Geometry check sheet. Reference: the model listing, model coordinates, mm. Face numbers are marked on the shaded views. A direction names the side the tool comes from. Round coordinates to 2 decimals unless told otherwise and drop trailing zeros. Write each loop counter-clockwise with the first axis right and the second up, starting at its lowest first coordinate (ties: lowest second). Pieces come first, ordered by that corner, then holes. Notation, with made-up numbers: M -8,77 L 12,77 A17 cw 12,105 Z; hole C -17,76.25 d11. An arc over 180 degrees is marked long. Put each result on its own line as item: value. Start each with the question number.
(1) Section check C-C on y = -9. Record the cut outline in (x, z) (3 decimals), then the cut area to 3 significant figures.
(2) Material ranges on probe 1 along Y at (x, z) = (16.5, 1.7); probe 2 along Y at (x, z) = (25.5, 2.95); probe 3 along Y at (x, z) = (29, 2), recorded low to high.
(3) Section check A-A on x = 17.5. Record the cut outline in (y, z) (1 decimal).
(4) Gauge pin test, flat ends, axial feed: pin 1 (1.6 mm diameter, centred on x = 22, z = 1.5, fed in from +Y); pin 2 (1.6 mm diameter, centred on x = -13.5, y = 16.5, fed in from -Z). Record the tip position at first contact, or that the pin passes through.
(5) Section check B-B on y = 6.35. Record the cut outline in (x, z) (3 decimals).
(6) Section check D-D on x = 10.5. Record the cut outline in (y, z) (3 decimals).
(7) Mould release check, pull along Y, two halves, no side actions. Record for the marked faces 4, 5 and 6: pulls with the +Y half, pulls with the -Y half, needs draft (parallel to the pull), parting line crosses it, or undercut.
(8) Tool access check on the marked faces 1, 2 and 3. Record the directions out of +Z, -Z, +X, -X, +Y, -Y that give a thin tool (end or side, any length) a straight path to the whole face; none if there is none.
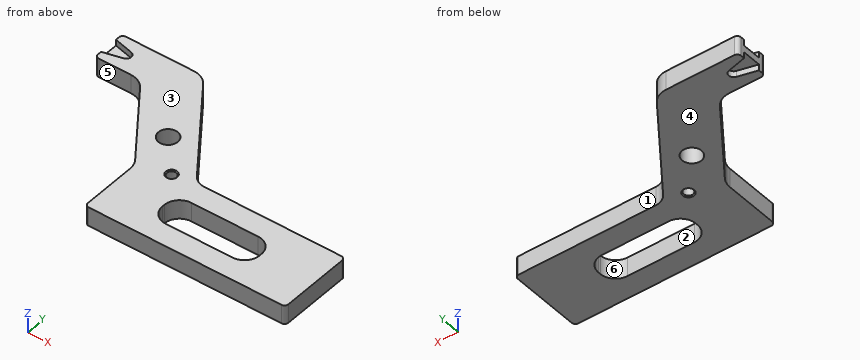
Autodesk Inventor part; units mm, degrees
ref_plane "Work Plane1" through (0, 0, 1.5875) normal (0, 0, 1) x (1, 0, 0)
ref_plane "YZ Plane" through (0, 0, 0) normal (1, 0, 0) x (0, 1, 0)
sketch "Sketch1" plane through (0, 0, 0) normal (0, 0, 1) x (1, 0, 0)
  line L0 (-20.447, 0) -> (20.447, 0)
  line L1 (0, -17.526) -> (0, 25.146)
  line L2 (14.605, -11.43) -> (-14.605, -11.43)
  line L3 (-14.605, -11.43) -> (-14.605, 19.05)
  line L4 (-14.605, 19.05) -> (14.605, 19.05)
  line L5 (14.605, 19.05) -> (14.605, -11.43)
  line L6 (-14.605, 16.6688) -> (-14.605, 19.05)
  point P0 (0, 0)
  dimension "d0" = 29.21
  dimension "d1" = 30.48
  dimension "d2" = 14.605
  dimension "d232" = 19.05
extrude "Extrusion2" add sketch "Sketch1" along normal blind 3.175
sketch "Sketch2" plane through (0, 0, 3.175) normal (0, 0, 1) x (1, 0, 0)
  line L0 (-14.605, -11.43) -> (-14.605, 19.05)
  line L1 (-14.605, 17.78) -> (-11.43, 16.9862)
  line L2 (-11.43, 16.9862) -> (-11.43, 15.3987)
  line L3 (-11.43, 15.3987) -> (-14.605, 14.605)
  line L4 (-14.605, 17.78) -> (-14.605, 14.605)
  line L5 (-14.605, 17.78) -> (-14.605, 19.05)
  arc A0 (-11.43, 15.3987) -> (-11.43, 16.9862) centre (-11.6284, 16.1925) ccw
  point P0 (0, 0)
  dimension "d21" = 3.175
  dimension "d22" = 1.5875
  dimension "d23" = 1.27
  dimension "d66" = 3.175
extrude "Extrusion3" cut sketch "Sketch2" against normal blind 1.016
sketch "Sketch11" plane through (0, 0, 3.175) normal (0, 0, 1) x (1, 0, 0)
  line L0 (14.605, -11.43) -> (-14.605, -11.43)
  line L1 (14.605, 1.27) -> (14.605, 19.05)
  line L2 (-14.605, 13.335) -> (-6.985, 13.335)
  line L3 (-6.985, 13.335) -> (3.175, -0.8164)
  line L4 (10.795, -11.43) -> (-14.605, -11.43)
  line L5 (14.605, 19.05) -> (14.605, -11.43)
  line L6 (14.605, 1.27) -> (11.8393, 1.27)
  line L7 (11.8393, 1.27) -> (-0.9259, 19.05)
  line L8 (-0.9259, 19.05) -> (14.605, 19.05)
  line L9 (-14.605, 13.335) -> (-14.605, -11.43)
  line L10 (3.175, -0.8164) -> (3.175, -11.43)
  point P0 (0, 0)
  point P1 (0, -11.43)
  dimension "d220" = 7.62
  dimension "d221" = 25.4
  dimension "d226" = 12.7
  dimension "d230" = 8.255
  dimension "d263" = 7.62
  dimension "d264" = 54.324
extrude "Extrusion10" cut sketch "Sketch11" against normal through all
sketch "Sketch12" plane through (0, 0, 3.175) normal (0, 0, 1) x (1, 0, 0)
  line L0 (-14.605, 19.05) -> (14.605, 19.05)
  line L1 (-14.605, -11.43) -> (-14.605, 19.05)
  line L2 (-0.2249, 19.05) -> (-2.4073, 19.05)
  line L3 (-0.2419, 3.9428) -> (6.4638, 8.7572)
  line L4 (-0.2419, 3.9428) -> (3.111, 6.35)
  line L5 (3.111, 6.35) -> (6.4638, 8.7572)
  line L6 (-6.985, 13.335) -> (3.175, -0.8164)
  line L7 (11.8393, 1.27) -> (-0.9259, 19.05)
  line L8 (0, 25.146) -> (0, -17.526)
  line L9 (-20.447, 0) -> (20.447, 0)
  point P0 (-14.605, 14.605)
  point P1 (10.795, -11.43)
  dimension "d231" = 6.35
hole "Hole9" at (3.111, 6.35, 3.175) direction (0, 0, -1) diameter 3.2512 end through all
sketch "Sketch16" plane through (14.605, -11.43, 3.175) normal (1, 0, 0) x (0, 0, -1)
  line L0 (3.175, 12.7) -> (0, 12.7)
  line L1 (0, 12.7) -> (0, 0)
  line L2 (3.175, 12.7) -> (3.175, 0)
  line L3 (3.175, 0) -> (0, 0)
  line L4 (0, 12.7) -> (3.175, 12.7)
  line L5 (3.175, 12.7) -> (3.175, 0)
  line L6 (3.175, 0) -> (0, 0)
  line L7 (0, 0) -> (0, 12.7)
extrude "Extrusion14" add sketch "Sketch16" along normal blind 22.098
hole "Hole14-Orig threaded Tscrew hole" [suppressed]
sketch "Sketch17" plane through (0, 0, 0) normal (0, 0, 1) x (1, 0, 0)
  circle A0 centre (8.1788, 0.635) radius 0.7937
  circle A1 centre (3.111, 6.35) radius 1.6256
  point P0 (0, 0)
  dimension "d235" = 1.5875
  dimension "d237" = 8.1788
  dimension "d238" = 5.0678
  dimension "d239" = 5.715
hole "Hole16" at (8.1788, 0.635, 0) direction (0, 0, 1) diameter 1.5748 end through all countersink diameter 1.905 countersink angle 90
fillet "Fillet9" radius 3.175 3 edges at (-0.9259, 19.05, 1.5875) (-6.985, 13.335, 1.5875) (3.175, -0.8164, 1.5875)
fillet "Fillet10" radius 0.635 2 edges at (-14.605, 19.05, 1.5875) (-14.605, 13.335, 1.5875)
ref_plane "Work Plane1" through (0, 0, 1.5875) normal (0, 0, 1) x (1, 0, 0)
mirror "Mirror1" about plane through (0, 0, 1.5875) normal (0, 0, 1) of "Extrusion3"
sketch "Sketch18" plane through (0, 0, 0) normal (0, 0, 1) x (1, 0, 0)
  line L0 (-13.97, 19.05) -> (-2.5549, 19.05)
  line L1 (-13.97, 13.335) -> (-8.6141, 13.335)
  line L2 (-14.605, 14.605) -> (-14.605, 17.78)
  line L3 (11.8393, 1.27) -> (0.0242, 17.7267)
  line L4 (-6.0349, 12.0117) -> (2.5791, 0.0135)
  circle A0 centre (3.111, 6.35) radius 1.6256
  circle A1 centre (8.1788, 0.635) radius 0.7874
  line L5 (-14.605, 19.05) -> (-0.9259, 19.05)
  line L6 (-6.985, 13.335) -> (-14.605, 13.335)
  line L7 (-14.605, 13.335) -> (-14.605, 19.05)
  line L8 (2.6983, -0.1524) -> (-6.985, 13.335)
  line L9 (-0.9259, 19.05) -> (7.3914, 7.4652)
  line L10 (7.3914, -0.1524) -> (2.6983, -0.1524)
  line L11 (7.3914, 7.4652) -> (7.3914, -0.1524)
  circle A2 centre (3.111, 6.35) radius 1.6256
  line L12 (-14.605, 17.78) -> (-14.605, 18.415)
  point P0 (10.8892, 2.5933)
  point P1 (9.8449, -10.1067)
  point P2 (10.795, -11.43)
  point P3 (6.985, -6.1232)
  dimension "d251" = 13.6791
  dimension "d252" = 5.715
  dimension "d253" = 7.62
  dimension "d254" = 14.2613
  dimension "d255" = 7.6176
  dimension "d256" = 4.6931
  dimension "d257" = 16.6035
  dimension "d258" = 21.9964
  dimension "d259" = 19.2024
  dimension "d260" = 12.7
  dimension "d261" = 17.716
fillet "Fillet11" radius 0.635 3 edges at (36.703, -11.43, 1.5875) (36.703, 1.27, 1.5875) (3.175, -11.43, 1.5875)
fillet "Fillet12" radius 2.54 1 edges at (11.8393, 1.27, 1.5875)
sketch "Sketch19" plane through (0, 0, 0) normal (0, 0, 1) x (1, 0, 0)
  line L0 (11.303, -2.3495) -> (27.559, -2.3495)
  line L1 (27.559, -2.3495) -> (27.559, -7.8105)
  line L2 (27.559, -7.8105) -> (11.303, -7.8105)
  line L3 (11.303, -7.8105) -> (11.303, -2.3495)
  line L4 (27.559, -5.08) -> (11.303, -5.08) construction
  line L5 (19.431, -2.3495) -> (19.431, -7.8105) construction
  line L6 (36.703, -10.795) -> (36.703, 0.635) construction
  line L7 (36.068, -11.43) -> (3.81, -11.43) construction
  point P0 (0, 0)
  dimension "d267" = 16.256
  dimension "d268" = 5.461
  dimension "d269" = 6.35
  dimension "d274" = 19.431
extrude "Extrusion15" cut sketch "Sketch19" along normal through all
fillet "Fillet13" radius 2.54 4 edges at (11.303, -7.8105, 1.5875) (11.303, -2.3495, 1.5875) (27.559, -7.8105, 1.5875) (27.559, -2.3495, 1.5875)
ref_plane "Work Plane2" through (0, -5.0927, 0) normal (0, 1, 0) x (-1, 0, 0)
chamfer "Chamfer9" distance 0.1651 angle 45 1 edges at (8.1788, -0.1524, 3.175)
equation "\"d2\" = 0.5 * d0"
properties part number "J002859" material "STAINLESS STEEL, 303"
Answers follow:
1. outline: M 3.175,0 L 36.703,0 L 36.703,3.175 L 3.175,3.175 Z
1. area: 106 mm^2
2. probe 1: y = -11.43 to -7.81, -2.35 to 1.27
2. probe 2: y = -11.43 to -7.76, -2.4 to 1.27
2. probe 3: y = -11.43 to 1.27
3. outline: M -11.4,0 L -7.8,0 L -7.8,3.2 L -11.4,3.2 Z; M -2.3,0 L 1.3,0 L 1.3,3.2 L -2.3,3.2 Z
4. pin 1: stops at y = 1.27
4. pin 2: stops at z = 1.02
5. outline: M -1.97,0 L 1.485,0 L 1.485,3.175 L -1.97,3.175 Z; M 4.737,0 L 8.192,0 L 8.192,3.175 L 4.737,3.175 Z
6. outline: M -11.43,0 L 3.135,0 L 3.135,3.175 L -11.43,3.175 Z
7. face 4: needs draft
7. face 5: pulls with the -Y half
7. face 6: undercut
8. face 1: +Z, -Z, +X, +Y
8. face 2: +Z, -Z
8. face 3: +Z, +X, -X, +Y, -Y
